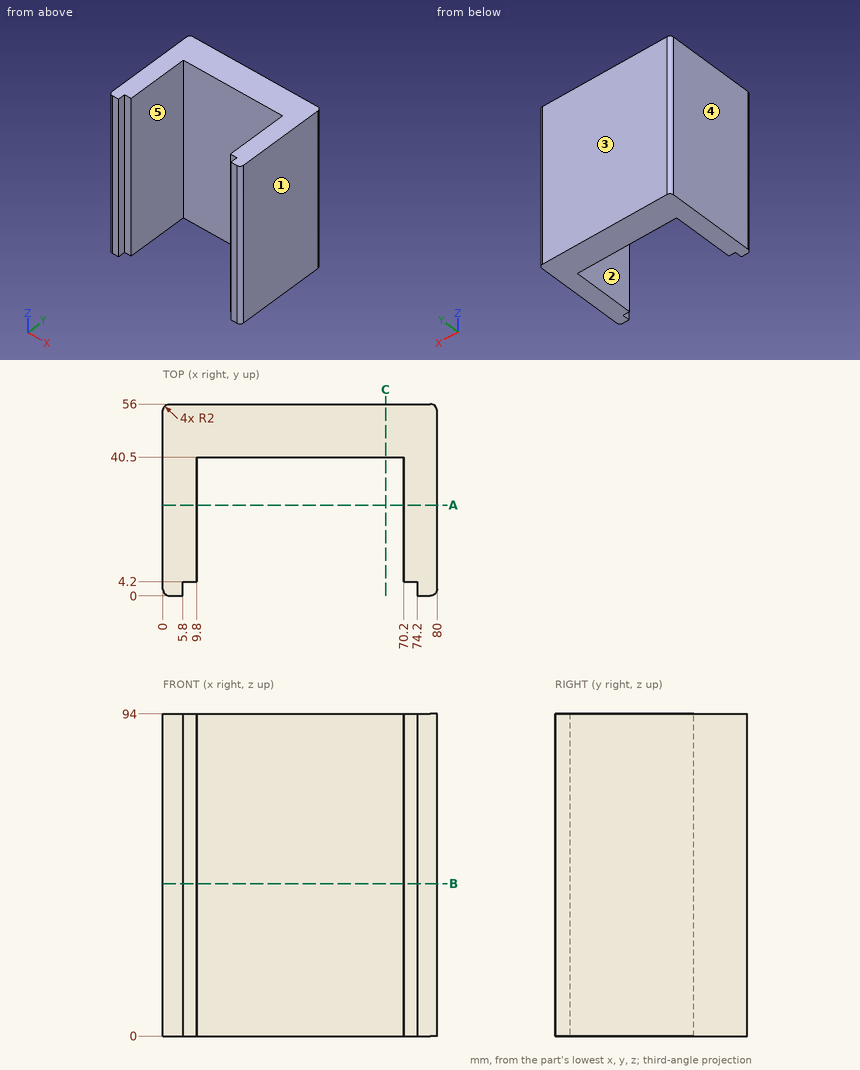
The drawing under review shows one solid part. Ordinate dimensions are in mm from its lowest x, y, z. A direction names the side the tool comes from. Coordinates: 2 decimals unless noted, no trailing zeros. Order: outer loops, then holes, each group sorted by start corner. A loop starts at its lowest first (then second) coordinate and runs counter-clockwise, first axis right, second up. Notation, with made-up numbers: M 1.5,22 L 27.5,22 A22 cw 27.5,33 Z; hole C 68.5,78.25 d7. An arc over 180 degrees is marked long. One line per question, with ' | ' between items.
(1) Machinability: for the marked faces 1 and 2, which of the approach directions +Z, -Z, +X, -X, +Y, -Y give a long, thin tool a straight path to every point of the face, cutting with its end or side? Answer none if there is none.
Geometry results:
face 1: +Z, -Z, +X, +Y, -Y | face 2: +Z, -Z, -Y
(2) Insertion check: pin 1 (12 mm diameter, centred on x = 42, z = 29.5, fed in from -Y); pin 2 (3 mm diameter, centred on x = 72.5, z = 42, fed in from -Y). Each pin has a flat end and moves straight along its axis. Give the tip position at first contact, or say it passes through.
Geometry results:
pin 1: stops at y = 40.5 | pin 2: stops at y = 4.2
(3) Add section A-A, the plane y = 26.5. Write out the cut boundary in (x, z), then the cut area to 3 significant figures.
Geometry results:
outline: M 0,0 L 9.8,0 L 9.8,94 L 0,94 Z; M 70.2,0 L 80,0 L 80,94 L 70.2,94 Z | area: 1,840 mm²
(4) Add section B-B, the plane z = 44.5. Write out the cut boundary in (x, y).
Geometry results:
outline: M 0,2 A2 ccw 2,0 L 5.8,0 L 5.8,4.2 L 9.8,4.2 L 9.8,40.5 L 70.2,40.5 L 70.2,4.2 L 74.2,4.2 L 74.2,0 L 78,0 A2 ccw 80,2 L 80,54 A2 ccw 78,56 L 2,56 A2 ccw 0,54 Z
(5) Add section C-C, the plane x = 65. Write out the cut boundary in (y, z).
Geometry results:
outline: M 40.5,0 L 56,0 L 56,94 L 40.5,94 Z
(6) For probe 1 along X at (y, z) = (24, 67); probe 2 along Y at (x, z) = (51, 17); probe 3 along Y at (x, z) = (72.5, 83.5), list the stretches that pass through material, from the lowest coordinate up. Write a range as from..to.
Geometry results:
probe 1: x = 0..9.8, 70.2..80 | probe 2: y = 40.5..56 | probe 3: y = 4.2..56
(7) The part is to be moulded in two halves that separate along X. For the marked faces 3, 4 and 5, say which applies: +X half, -X half, draft (parallel to the pull), parting line (faces both ways), or undercut.
Geometry results:
face 3: draft | face 4: -X half | face 5: undercut
